Check sheet for the modelled part. Datum: model origin and axes. Units: mm. A direction names the side the tool comes from. Coordinates: 2 decimals unless noted, no trailing zeros. Write each loop counter-clockwise with the first axis right and the second up, starting at its lowest first coordinate (ties: lowest second). Pieces come first, ordered by that corner, then holes. Notation, with made-up numbers: (-19.75, -26.5) - (1.25, -26.5) arc R10 ccw to (1.25, -10.5) - close; hole circle Ø8 at (-24.5, 85.5). An arc over 180 degrees is marked (long way). Write each question's results on one line, items separated by ' | '.
from build123d import *

# Parameters (mm, degrees)
F2_SIZE = 0.99999


# Not quite as in the source:
# - a fillet or chamfer is up to 0.001 mm smaller than in the source, because OpenCascade refuses the exact size


with BuildPart() as f1:
    # F0 (on Right) → F1 (revolve)
    with BuildSketch(Plane.YZ):
        Polygon((0, 5), (0, 0), (635, 0), (635, 5), (624, 5), (624, 8), (54, 8), (54, 6), (15, 6), (15, 5), align=None)
    revolve(axis=Axis((0, 344.1624132916, 0), (0, 1, 0)))

    # F2 (size 1 in the source; OpenCascade refuses exactly that, so slightly less here)
    f2_edges = [f1.edges().sort_by_distance(p)[0] for p in [
        (0, 0, -5),
        (0, 15, -6),
        (0, 635, -5),
    ]]
    chamfer(f2_edges, length=F2_SIZE)


solid = f1.part
1. Go/stop test with flat-tipped pins: pin 1 (4 mm diameter, centred on x = -4, y = 334.5, fed in from -Z); pin 2 (1.5 mm diameter, centred on y = 155.5, z = -2.5, fed in from -X); pin 3 (3 mm diameter, centred on y = 256.5, z = 5, fed in from -X). Record where each tip stops, or that it passes through.
Values follow:
pin 1: stops at z = -7.75 | pin 2: stops at x = -7.81 | pin 3: stops at x = -7.19
2. Sectioned sample at C-C (y = 291.5). Record the cut outline in (x, z), then the cut area to 3 significant figures.
Values follow:
outline: circle Ø16 at (0, 0) | area: 201 mm^2
3. Access from +Z, -Z, +X, -X, +Y, -Y to the whole of each face (thin tool, end or side, straight path). Record for faces 1 (the flat face through (-5.2, 624, 0.1)), 2 (the cylindrical face through (-7.81, 335.01, -1.73)), 3 (the cylindrical face through (-4.88, 7.9, -1.08)).
Values follow:
face 1: +Y | face 2: +Y, -Y | face 3: -Y
4. Material ranges on L1, parallel to X at y = 380, z = 1.25; L2, parallel to X at y = 295, z = -0.25; L3, parallel to Z at x = 0.5, y = 455, recorded low to high. Write a range as [from, to].
Values follow:
L1: x = [-7.9, 7.9] | L2: x = [-8, 8] | L3: z = [-7.98, 7.98]
